```python
from build123d import *

# Parameters (mm, degrees)
SKETCH_1_W          = 145
SKETCH_1_H          = 59.3
EXTRUDE_1_DEPTH     = 4
SKETCH_2_R          = 2.1
CUT_EXTRUDE_1_DEPTH = 4
SKETCH_3_R          = 1.6
CUT_EXTRUDE_2_DEPTH = 4
FILLET_1_R          = 2
CUT_EXTRUDE_3_DEPTH = 5


with BuildPart() as part:
    # 草图1 → 凸台-拉伸1 (new body)
    with BuildSketch(Plane.XY):
        Rectangle(SKETCH_1_W, SKETCH_1_H)
    extrude(amount=EXTRUDE_1_DEPTH)

    # 草图2 → 切除-拉伸1 (cut)
    with BuildSketch(Plane.XY.offset(4)):
        with Locations((-67.5, 21.65)):
            Circle(SKETCH_2_R)
        with Locations((67.5, 21.65)):
            Circle(SKETCH_2_R)
        with Locations((67.5, -3.35)):
            Circle(SKETCH_2_R)
        with Locations((-67.5, -3.35)):
            Circle(SKETCH_2_R)
        with Locations((-47.5, 21.65)):
            Circle(SKETCH_2_R)
        with Locations((47.5, 21.65)):
            Circle(SKETCH_2_R)
        with Locations((47.5, -3.35)):
            Circle(SKETCH_2_R)
        with Locations((-47.5, -3.35)):
            Circle(SKETCH_2_R)
    extrude(amount=-CUT_EXTRUDE_1_DEPTH, mode=Mode.SUBTRACT)

    # 草图3 → 切除-拉伸2 (cut)
    with BuildSketch(Plane.XY.offset(4)):
        with Locations((-40, 4.25)):
            Circle(SKETCH_3_R)
        with Locations((40, 4.25)):
            Circle(SKETCH_3_R)
        with Locations((40, -25.75)):
            Circle(SKETCH_3_R)
        with Locations((-40, -25.75)):
            Circle(SKETCH_3_R)
    extrude(amount=-CUT_EXTRUDE_2_DEPTH, mode=Mode.SUBTRACT)

    # 圆角1
    fillet_1_edges = [part.edges().sort_by_distance(p)[0] for p in [
        (72.5, -29.65, 2),
        (-72.5, -29.65, 2),
        (-72.5, 29.65, 2),
        (72.5, 29.65, 2),
    ]]
    fillet(fillet_1_edges, radius=FILLET_1_R)

    # 草图4 → 切除-拉伸3 (cut)
    with BuildSketch(Plane.XY.offset(4)):
        with BuildLine():
            Line((-28.5, 21.65), (-28.5, -21.65))
            ThreePointArc((-28.5, -21.65), (-31.5, -24.65), (-34.5, -21.65))
            Line((-34.5, -21.65), (-34.5, 21.65))
            ThreePointArc((-34.5, 21.65), (-31.5, 24.65), (-28.5, 21.65))
        make_face()
        with BuildLine():
            Line((-19.5, 21.65), (-19.5, -21.65))
            ThreePointArc((-19.5, -21.65), (-22.5, -24.65), (-25.5, -21.65))
            Line((-25.5, -21.65), (-25.5, 21.65))
            ThreePointArc((-25.5, 21.65), (-22.5, 24.65), (-19.5, 21.65))
        make_face()
        with BuildLine():
            Line((-10.5, 21.65), (-10.5, -21.65))
            ThreePointArc((-10.5, -21.65), (-13.5, -24.65), (-16.5, -21.65))
            Line((-16.5, -21.65), (-16.5, 21.65))
            ThreePointArc((-16.5, 21.65), (-13.5, 24.65), (-10.5, 21.65))
        make_face()
        with BuildLine():
            Line((-1.5, 21.65), (-1.5, -21.65))
            ThreePointArc((-1.5, -21.65), (-4.5, -24.65), (-7.5, -21.65))
            Line((-7.5, -21.65), (-7.5, 21.65))
            ThreePointArc((-7.5, 21.65), (-4.5, 24.65), (-1.5, 21.65))
        make_face()
        with BuildLine():
            Line((7.5, 21.65), (7.5, -21.65))
            ThreePointArc((7.5, -21.65), (4.5, -24.65), (1.5, -21.65))
            Line((1.5, -21.65), (1.5, 21.65))
            ThreePointArc((1.5, 21.65), (4.5, 24.65), (7.5, 21.65))
        make_face()
        with BuildLine():
            Line((16.5, 21.65), (16.5, -21.65))
            ThreePointArc((16.5, -21.65), (13.5, -24.65), (10.5, -21.65))
            Line((10.5, -21.65), (10.5, 21.65))
            ThreePointArc((10.5, 21.65), (13.5, 24.65), (16.5, 21.65))
        make_face()
        with BuildLine():
            Line((25.5, 21.65), (25.5, -21.65))
            ThreePointArc((25.5, -21.65), (22.5, -24.65), (19.5, -21.65))
            Line((19.5, -21.65), (19.5, 21.65))
            ThreePointArc((19.5, 21.65), (22.5, 24.65), (25.5, 21.65))
        make_face()
        with BuildLine():
            Line((34.5, 21.65), (34.5, -21.65))
            ThreePointArc((34.5, -21.65), (31.5, -24.65), (28.5, -21.65))
            Line((28.5, -21.65), (28.5, 21.65))
            ThreePointArc((28.5, 21.65), (31.5, 24.65), (34.5, 21.65))
        make_face()
    extrude(amount=-CUT_EXTRUDE_3_DEPTH, mode=Mode.SUBTRACT)


solid = part.part
```
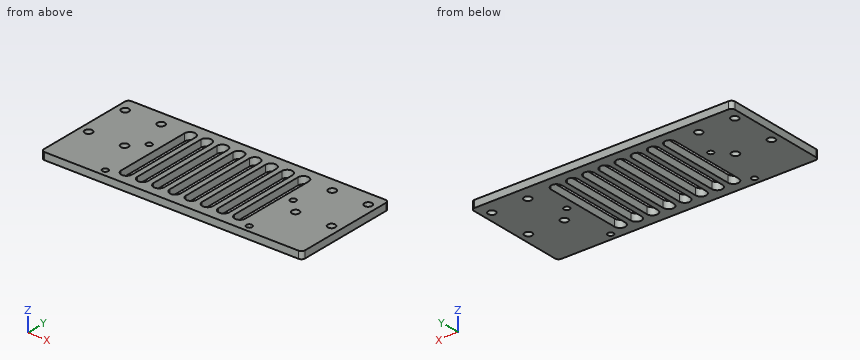
The listing builds one solid part. Answer for the finished solid, in the listing's coordinates (mm). Give positions to 0.01 mm unless a question says otherwise; leave off trailing zeros. Order: outer loops, then holes, each group sorted by start corner. A loop starts at its lowest first (then second) coordinate and runs counter-clockwise, first axis right, second up. Notation, with made-up numbers: (11, 48.25) -> (41, 48.25) arc R3 cw to (41, 53.25) -> close; hole circle Ø8 at (39.5, 42.5). An arc over 180 degrees is marked (long way). Write each question's results on one line, items separated by ' | '.
Q1. The part is cut by section C-C, the plane y = 4.25. State how many separate pieces and enclosed holes the cut face has, and give its area (3 significant figures).
Checked values:
separate pieces: 11 | enclosed holes: 0 | area: 362 mm^2
Q2. Straight lines are drawn through the part: probe 1 along Y at (x, z) = (47.5, 1.2); probe 2 along Y at (x, z) = (-22.5, 1.65); probe 3 along Y at (x, z) = (-48.5, 2.3). For each, find the intervals that lie inside material, in ascending order. Write a range as from..to.
Checked values:
probe 1: y = -29.65..-5.45, -1.25..19.55, 23.75..29.65 | probe 2: y = -29.65..-24.65, 24.65..29.65 | probe 3: y = -29.65..-5.2, -1.5..19.8, 23.5..29.65
Q3. This flat-tipped pin is pushed along its axis until it touches: P1, Ø1.9, axis at x = -40, y = 4.25, coming from the -Z side. Where does it stop, or does it pass through?
Checked values:
P1: passes through
Q4. The part is cut by section A-A, the plane x = -4.5. Give the vertices of the cut face in (y, z).
Checked values:
outline: (-29.65, 0) -> (-24.65, 0) -> (-24.65, 4) -> (-29.65, 4) -> close; (24.65, 0) -> (29.65, 0) -> (29.65, 4) -> (24.65, 4) -> close
Q5. The part is cut by section B-B, the plane x = -47.5. Give the vertices of the cut face in (y, z), and give its area (3 significant figures).
Checked values:
outline: (-29.65, 0) -> (-5.45, 0) -> (-5.45, 4) -> (-29.65, 4) -> close; (-1.25, 0) -> (19.55, 0) -> (19.55, 4) -> (-1.25, 4) -> close; (23.75, 0) -> (29.65, 0) -> (29.65, 4) -> (23.75, 4) -> close | area: 204 mm^2
